```python
from build123d import *

# Parameters (mm, degrees)
EXTRUDE_DEPTH  = 14
SKETCH_R       = 15
SKETCH_R_2     = 14
PAD_DEPTH      = 20
PAD_DEPTH_BACK = 20
PAD001_DEPTH   = 0.5
PAD002_DEPTH   = 0.5
POCKET_DEPTH   = 7.001
SKETCH012_R    = 14
SKETCH005_R    = 15


with BuildPart() as extrude_body:
    # Sketch009 (on Face1 of CopyCut001) → Extrude (new body)
    with BuildSketch(Plane(origin=(0, 0, -6), x_dir=(1, 0, 0), z_dir=(0, 0, -1))):
        with BuildLine():
            ThreePointArc((-8, -6.408003), (10.25, 0), (-8, 6.408003))
            Line((-8, 6.408003), (-8, -6.408003))
        make_face()
        with BuildLine():
            ThreePointArc((-7, -6.046693), (9.25, 0), (-7, 6.046693))
            Line((-7, -6.046693), (-7, 6.046693))
        make_face(mode=Mode.SUBTRACT)
    extrude(amount=EXTRUDE_DEPTH)


with BuildPart() as body:
    # Sketch → Pad (new body, two sides)
    with BuildSketch(Plane.XY) as pad_sk:
        Circle(SKETCH_R)
        Circle(SKETCH_R_2, mode=Mode.SUBTRACT)
    extrude(amount=PAD_DEPTH)
    extrude(pad_sk.sketch, amount=-PAD_DEPTH_BACK)

    # Sketch002 (on DatumPlane) → Pad001 (join)
    with BuildSketch(Plane.XY.offset(19.5)):
        Polygon((13.5, 0), (14, 0), (14, 0.5), align=None)
    extrude(amount=PAD001_DEPTH)

    # Sketch003 (on DatumPlane) → Pad002 (join)
    with BuildSketch(Plane(origin=(0, 0, -19.5), x_dir=(1, 0, 0), z_dir=(0, 0, -1))):
        Polygon((13.5, 0), (14, 0), (14, 0.5), align=None)
    extrude(amount=PAD002_DEPTH)

    # Sketch010 (on Face1 of CopyExtrude001) → Pocket (cut, through all)
    with BuildSketch(Plane(origin=(-8, 0, 0), x_dir=(0, -1, 0), z_dir=(-1, 0, 0))):
        Polygon((0, 3), (2.828427, 5.828427), (0, 8.656854), (-2.828427, 5.828427), align=None)
    extrude(amount=POCKET_DEPTH, mode=Mode.SUBTRACT)


with BuildPart() as loft001:
    # Sketch007 (on Face1 of CopyLoft001) → Loft001 section 0
    with BuildSketch(Plane(origin=(0, 0, -6), x_dir=(1, 0, 0), z_dir=(0, 0, -1))):
        with BuildLine():
            ThreePointArc((-7, -6.046693), (9.25, 0), (-7, 6.046693))
            Line((-7, 6.046693), (-7, -6.046693))
        make_face()
    # Sketch012 (on Face1 of CopyLoft002) → Loft001 section 1
    with BuildSketch(Plane.XY.offset(13)):
        Circle(SKETCH012_R)
    loft()


with BuildPart() as fusion:
    # Sketch005 (on DatumPlane) → Loft section 0
    with BuildSketch(Plane.XY.offset(13)):
        Circle(SKETCH005_R)
    # Sketch004 (on DatumPlane) → Loft section 1
    with BuildSketch(Plane(origin=(0, 0, -6), x_dir=(1, 0, 0), z_dir=(0, 0, -1))):
        with BuildLine():
            ThreePointArc((-8, -6.408003), (10.25, 0), (-8, 6.408003))
            Line((-8, 6.408003), (-8, -6.408003))
        make_face()
    loft()

    # Cut: cut Loft001
    add(loft001.part, mode=Mode.SUBTRACT)

    # Fusion: union Extrude body, Body
    add(extrude_body.part)
    add(body.part)


solid = fusion.part
```
Geometry: final body of the model. Coordinates: model frame, mm. A direction names the side the tool comes from. Give positions to 0.01 mm unless a question says otherwise; leave off trailing zeros. Loops run counter-clockwise (first coordinate to the right, second up) from the corner with the lowest first, then second, coordinate; pieces in that order, holes last. Notation, with made-up numbers: (63.25, -11) -> (95.25, -11) arc R27 cw to (95.25, 11) -> close; hole circle Ø8 at (-14, -19). An arc over 180 degrees is marked (long way). Use CSV: the item, a comma, the result in double quotes.
(1) Access query for faces 3 (the face through (-14.347, 1.394, 7.262)), 4 (the face through (-7, 0, -13)), 5 (the face through (-8, 0, -13)). Directions: +Z, -Z, +X, -X, +Y, -Y. A direction counts if a zero-diameter tool reaches every point of the face in a straight line with its end or side. Return the directions, or none.
From the geometry:
face 3,"-X"
face 4,"+Z, -Z"
face 5,"-Z"
(2) Ray query, line 1 along Y through (x, z) = (0, -11); line 2 along Y through (x, z) = (0, 15); line 3 along X through (y, z) = (6, -14.5). Return the intervals inside material, ascending. Write a range as [from, to].
From the geometry:
line 1,"[-15, -14], [-10.25, -9.25], [9.25, 10.25], [14, 15]"
line 2,"[-15, -14], [14, 15]"
line 3,"[-13.75, -12.65], [-8, -7], [7.04, 8.31], [12.65, 13.75]"
(3) First-contact query: P1, Ø2, axis at y = -1.5, z = -6.5, coming from the -X side; P2, Ø5, axis at y = 8, z = -5.5, coming from the -X side; P3, Ø12, axis at y = 10.5, z = 4.5, coming from the +X side; P4, Ø1.5, axis at x = -3.5, y = 5.5, coming from the -Z side. Flat tips, straight axial feed; report the tip coordinate or a pass-through.
From the geometry:
P1,"x = -14.99"
P2,"x = -13.96"
P3,"x = 14.31"
P4,"through"
(4) Cut plane A-A (z = -15). Output: boundary loops of the cut face in (x, y), plus the area to 3 significant figures.
From the geometry:
outline,"circle Ø30 at (0, 0); (-8, -6.41) arc R10.25 ccw (long way) to (-8, 6.41) -> close; hole circle Ø28 at (0, 0); hole (-7, -6.05) arc R9.25 ccw (long way) to (-7, 6.05) -> close"
area,"151 mm^2"
(5) Pull-direction query (Z, two-part tool) for faces 1 (the face through (10.244, 0.354, -12.902)), 2 (the face through (-14.3, -1.4, 4.4)); classes: released by +Z, released by -Z, zero draft, split by the parting line, or undercut.
From the geometry:
face 1,"zero draft"
face 2,"undercut"
(6) Cut plane B-B (z = 17.5). Output: boundary loops of the cut face in (x, y).
From the geometry:
outline,"circle Ø30 at (0, 0); hole circle Ø28 at (0, 0)"
